Design review of the part built by this model. Coordinates are the model's own, in mm. A direction names the side the tool comes from. Give positions to 0.01 mm unless a question says otherwise; leave off trailing zeros. Write each loop counter-clockwise with the first axis right and the second up, starting at its lowest first coordinate (ties: lowest second). Pieces come first, ordered by that corner, then holes.
```python
from build123d import *

# Parameters (mm, degrees)
F0_R     = 58.94491
F0_R_2   = 21.394651
F1_DEPTH = 25
F2_R     = 7.799399
F2_R_2   = 13.108155
F3_DEPTH = 25
F4_DEPTH = 25
F5_W     = 10.734647
F5_H     = 32.95438
F6_DEPTH = 25


with BuildPart() as f1:
    # F0 (on Top) → F1 (new body)
    with BuildSketch(Plane.XY):
        with Locations((-34.007099, 3.729807)):
            Circle(F0_R)
        with Locations((-7.240221, 0)):
            Circle(F0_R_2, mode=Mode.SUBTRACT)
    extrude(amount=F1_DEPTH)

    # F2 (on face) → F3 (join)
    with BuildSketch(Plane.XY.offset(25)):
        with Locations((-66.981934, -11.72878)):
            Circle(F2_R)
        with Locations((-55.42469, 36.005322)):
            Circle(F2_R_2)
    extrude(amount=F3_DEPTH)

    # F2 (on face) → F4 (join)
    with BuildSketch(Plane.XY.offset(25)):
        with Locations((-66.981934, -11.72878)):
            Circle(F2_R)
    extrude(amount=F4_DEPTH)

    # F5 (on face) → F6 (join)
    with BuildSketch(Plane.XY.offset(25)):
        with Locations((-37.361666, 0)):
            Rectangle(F5_W, F5_H)
    extrude(amount=F6_DEPTH)


solid = f1.part
```
(1) Consider section C-C, the plane z = 38. Give the boundary of the cut face in (x, y), then the cut area to 3 significant figures.
Resolved:
outline: circle Ø15.6 at (-66.98, -11.73); circle Ø26.22 at (-55.42, 36.01); (-42.73, -16.48) - (-31.99, -16.48) - (-31.99, 16.48) - (-42.73, 16.48) - close
area: 1,080 mm2
(2) Tool access review of faces 4 (the face through (-31.994, 0, 37)), 5 (the face through (-42.729, 0, 37)), 6 (the face through (-59.78, -14.72, 37.33)), 7 (the face through (-37, -16.477, 37)): name each direction out of +Z, -Z, +X, -X, +Y, -Y from which nothing blocks a thin tool from reaching the whole face with its end or side.
Resolved:
face 4: +Z, +X, +Y, -Y
face 5: +Z, -Y
face 6: +Z
face 7: +Z, +X, -Y
(3) Consider section B-B, the plane x = -25. Give the boundary of the cut face in (y, z).
Resolved:
outline: (-54.52, 0) - (-11.93, 0) - (-11.93, 25) - (-54.52, 25) - close; (11.93, 0) - (61.98, 0) - (61.98, 25) - (11.93, 25) - close
(4) To check wall thickness, follow L1, parallel to Z at x = 15, y = -4.5; L2, parallel to X at y = 18.5, z = 24; L3, parallel to X at y = 12, z = 3. State the ranges of each line that lie inside material, in increasing order.
Resolved:
L1: z = 0 to 25
L2: x = -91.07 to -17.99, 3.51 to 23.06
L3: x = -92.37 to -24.95, 10.47 to 24.35
(5) Mouldability with a two-part tool opening along Y and no side actions: class faces 1 (the face through (-67, -12, 50)), 2 (the face through (12.523, -8.194, 12.325)), 3 (the face through (-92.895, 6.322, 12.325)) as pulls with the +Y half, pulls with the -Y half, needs draft (parallel to the pull), parting line crosses it, or undercut.
Resolved:
face 1: needs draft
face 2: undercut
face 3: parting line crosses it
(6) Consider section A-A, the plane y = 12. Give the boundary of the cut face in (x, z).
Resolved:
outline: (-92.37, 0) - (-24.95, 0) - (-24.95, 25) - (-31.99, 25) - (-31.99, 50) - (-42.73, 50) - (-42.73, 25) - (-92.37, 25) - close; (10.47, 0) - (24.35, 0) - (24.35, 25) - (10.47, 25) - close
(7) Consider section D-D, the plane x = -39.5. Give the boundary of the cut face in (y, z), then the cut area to 3 significant figures.
Resolved:
outline: (-54.96, 0) - (62.42, 0) - (62.42, 25) - (16.48, 25) - (16.48, 50) - (-16.48, 50) - (-16.48, 25) - (-54.96, 25) - close
area: 3,760 mm2
(8) Clearance check with flat-ended pins moving along their axes: P1, Ø2, axis at x = -37, z = 42.5, coming from the +Y side; P2, Ø1.5, axis at y = 36.5, z = 34, coming from the -X side; P3, Ø6, axis at x = -40, y = -40, coming from the +Z side. State where each tip first meets the part, or that it passes through.
Resolved:
P1: stops at y = 16.48
P2: stops at x = -68.53
P3: stops at z = 25
